```python
from build123d import *

# Parameters (mm, degrees)
F0_W     = 4.25
F0_H     = 2.8
F0_W_2   = 10.25
F0_H_2   = 15.6
F4_W     = 4.8
F4_H     = 8.5
F5_DEPTH = 15.6
F6_R     = 1.2
F7_DEPTH = 16.901


with BuildPart() as f1:
    # F0 (on Front) → F1 (revolve)
    with BuildSketch(Plane.XZ):
        with Locations((2.125, 1.4)):
            Rectangle(F0_W, F0_H)
        with Locations((9.375, 1.4)):
            Rectangle(F0_W_2, F0_H)
        with Locations((2.125, 10.6)):
            Rectangle(F0_W, F0_H_2)
    revolve(axis=Axis((0, 0, 8.798894), (0, 0, -1)))

    # F2 (on Front) → F3 (revolve, cut)
    with BuildSketch(Plane.XZ):
        Polygon((14.5, 2.8), (11.75, 2.8), (14.5, 0.5), align=None)
    revolve(axis=Axis((0, 0, 11.99575), (0, 0, 1)), mode=Mode.SUBTRACT)

    # F4 (on face) → F5 (cut, through all)
    with BuildSketch(Plane.XY.offset(18.4)):
        with Locations((4.8, 0)):
            Rectangle(F4_W, F4_H)
        with Locations((-4.8, 0)):
            Rectangle(F4_W, F4_H)
    extrude(amount=-F5_DEPTH, mode=Mode.SUBTRACT)

    # F6 (on face) → F7 (cut, through all)
    with BuildSketch(Plane(origin=(-2.4, 0, 0), x_dir=(0, -1, 0), z_dir=(-1, 0, 0))):
        with Locations((0, 15.2)):
            Circle(F6_R)
    extrude(amount=-F7_DEPTH, mode=Mode.SUBTRACT)


solid = f1.part
```
Verification items for the finished model (mm, model axes). A direction names the side the tool comes from. Give positions to 0.01 mm unless a question says otherwise; leave off trailing zeros. Order: outer loops, then holes, each group sorted by start corner. A loop starts at its lowest first (then second) coordinate and runs counter-clockwise, first axis right, second up. Notation, with made-up numbers: M 21.25,62 L 76.25,62 A22 cw 76.25,70 Z; hole C -34.75,30.5 d10. An arc over 180 degrees is marked long. Return JSON: item names as keys, results as strings. Group by question number.
1) Section check A-A on z = 15.2. Record the cut outline in (x, y), and give its area (3 significant figures).
2) Section check C-C on x = 0. Record the cut outline in (y, z).
3) Section check B-B on y = 0. Record the cut outline in (x, z).
4) Mould release check, pull along Y, two halves, no side actions. Record for faces 1 (the face through (11.37, 3.58, 2.66)), 2 (the face through (0, 0, 14)), 3 (the face through (2.4, 0, 11)), 4 (the face through (0.04, -4.25, 10.71)): pulls with the +Y half, pulls with the -Y half, needs draft (parallel to the pull), parting line crosses it, or undercut.
5) Access from +Z, -Z, +X, -X, +Y, -Y to the whole of each face (thin tool, end or side, straight path). Record for faces 5 (the face through (6.691, 12.864, 0.254)), 6 (the face through (-2.4, 0, 11)), 7 (the face through (-0.04, 4.25, 10.71)).
6) Scan lines: line 1 (Z direction, x = 0.4, y = 0); line 2 (Z direction, x = 9.25, y = -5.25); line 3 (X direction, y = 1.75, z = 8.25). Record each from-to range of solid material in increasing order.
7) Go/stop test with flat-tipped pins: pin 1 Ø3 at (y, z) = (-3.5, 9.5) entering from -X; pin 2 Ø7.5 at (y, z) = (-1, 11) entering from +X; pin 3 Ø2 at (y, z) = (0, 15.2) entering from -X; pin 4 Ø8 at (x, z) = (4.5, 5) entering from -Y. Record where each tip stops, or that it passes through.
Answer block:
{
 "1": {"outline": "M -2.4,-3.51 A4.25 ccw 2.4,-3.51 L 2.4,-1.2 L -2.4,-1.2 Z; M -2.4,1.2 L 2.4,1.2 L 2.4,3.51 A4.25 ccw -2.4,3.51 Z", "area": "27.0 mm^2"},
 "2": {"outline": "M -14.5,0 L 14.5,0 L 14.5,0.5 L 11.75,2.8 L 4.25,2.8 L 4.25,18.4 L -4.25,18.4 L -4.25,2.8 L -11.75,2.8 L -14.5,0.5 Z; hole C 0,15.2 d2.4"},
 "3": {"outline": "M -14.5,0 L 14.5,0 L 14.5,0.5 L 11.75,2.8 L 2.4,2.8 L 2.4,14 L -2.4,14 L -2.4,2.8 L -11.75,2.8 L -14.5,0.5 Z; M -2.4,16.4 L 2.4,16.4 L 2.4,18.4 L -2.4,18.4 Z"},
 "4": {"face 1": "parting line crosses it", "face 2": "undercut", "face 3": "needs draft", "face 4": "pulls with the -Y half"},
 "5": {"face 5": "+Z, -Z", "face 6": "+Z, -X, +Y, -Y", "face 7": "+Z, +Y"},
 "6": {"line 1": "z = 0 to 14, 16.4 to 18.4", "line 2": "z = 0 to 2.8", "line 3": "x = -2.4 to 2.4"},
 "7": {"pin 1": "stops at x = -2.4", "pin 2": "stops at x = 2.4", "pin 3": "passes through", "pin 4": "stops at y = -13.3"}
}
